```python
from build123d import *

# Parameters (mm, degrees)
BOSS_EXTRUDE1_DEPTH   = 14.2875
F_4_CLEARANCE_HOLE1_D = 3.2639
BOSS_EXTRUDE2_START   = 3.175
SKETCH6_R             = 3.175
SKETCH6_R_2           = 1.63195
BOSS_EXTRUDE2_DEPTH   = 3.175
FILLET1_R             = 3.175
F_2_CLEARANCE_HOLE2_D = 2.4384


with BuildPart() as part:
    # Sketch2 → Boss-Extrude1 (new, symmetric)
    with BuildSketch(Plane.XY):
        Polygon((-14.2875, 0), (-14.2875, 5.08), (-4.5, 5.08), (-4.5, 2.54), (4.5, 2.54), (4.5, 5.08), (14.2875, 5.08), (14.2875, 0), align=None)
    extrude(amount=BOSS_EXTRUDE1_DEPTH, both=True)

    # #4 Clearance Hole1 (through all)
    with Locations(Plane(origin=(0, 5.08, 0), x_dir=(1, 0, 0), z_dir=(0, 1, 0))):
        with Locations((-11.1125, 11.1125), (11.1125, -11.1125), (11.1125, 11.1125), (-11.1125, -11.1125)):
            Hole(F_4_CLEARANCE_HOLE1_D / 2)

    # Sketch6 → Boss-Extrude2 (add)
    # profile 1 of 4: a face of its own
    with BuildSketch(Plane.XZ.offset(BOSS_EXTRUDE2_START)):
        with Locations(Location((-11.1125, 11.1125, 0), (0, 0, 180))):
            Circle(SKETCH6_R)
        with Locations(Location((-11.1125, 11.1125, 0), (0, 0, 90))):
            Circle(SKETCH6_R_2, mode=Mode.SUBTRACT)
    # profile 2 of 4: a face of its own
    with BuildSketch(Plane.XZ.offset(BOSS_EXTRUDE2_START)):
        with Locations((11.1125, 11.1125)):
            Circle(SKETCH6_R)
        with Locations(Location((11.1125, 11.1125, 0), (0, 0, 90))):
            Circle(SKETCH6_R_2, mode=Mode.SUBTRACT)
    # profile 3 of 4: a face of its own
    with BuildSketch(Plane.XZ.offset(BOSS_EXTRUDE2_START)):
        with Locations((11.1125, -11.1125)):
            Circle(SKETCH6_R)
        with Locations(Location((11.1125, -11.1125, 0), (0, 0, 90))):
            Circle(SKETCH6_R_2, mode=Mode.SUBTRACT)
    # profile 4 of 4: a face of its own
    with BuildSketch(Plane.XZ.offset(BOSS_EXTRUDE2_START)):
        with Locations(Location((-11.1125, -11.1125, 0), (0, 0, 180))):
            Circle(SKETCH6_R)
        with Locations(Location((-11.1125, -11.1125, 0), (0, 0, 90))):
            Circle(SKETCH6_R_2, mode=Mode.SUBTRACT)
    extrude(amount=-BOSS_EXTRUDE2_DEPTH)

    # Fillet1
    fillet1_edges = [part.edges().sort_by_distance(p)[0] for p in [
        (-14.2875, 2.54, -14.2875),
        (-14.2875, 2.54, 14.2875),
        (14.2875, 2.54, -14.2875),
        (14.2875, 2.54, 14.2875),
    ]]
    fillet(fillet1_edges, radius=FILLET1_R - 0.0001)  # a hair under: the kernel refuses the full size

    # #2 Clearance Hole2 (through all)
    with Locations(Plane(origin=(0, 2.54, 0), x_dir=(1, 0, 0), z_dir=(0, 1, 0))):
        with Locations((-2.999999969, 5.999999938), (2.999999969, -5.999999938), (2.999999969, 5.999999938), (-2.999999969, -5.999999938)):
            Hole(F_2_CLEARANCE_HOLE2_D / 2)


solid = part.part
```
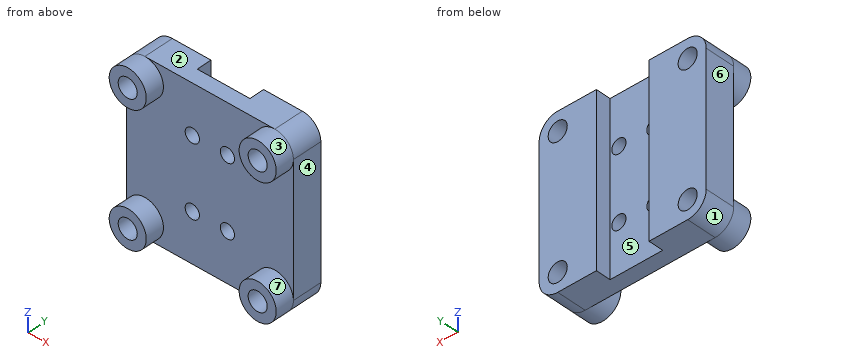
Check sheet for the modelled part. Datum: model origin and axes. Units: mm. Face numbers are marked on the shaded views. A direction names the side the tool comes from. Coordinates: 2 decimals unless noted, no trailing zeros. Write each loop counter-clockwise with the first axis right and the second up, starting at its lowest first coordinate (ties: lowest second). Pieces come first, ordered by that corner, then holes. Notation, with made-up numbers: M 30,9 L 79,9 A23 ccw 79,33 Z; hole C -29.75,-11 d9. An arc over 180 degrees is marked long. Write item = value, one per line. Start each with the question number.
1. Sectioned sample at A-A (y = -0.5). State how many separate pieces and enclosed holes the cut face has, then the cut area to 3 significant figures.
2. Thickness scan on probe 1 along Z at (x, y) = (-3, 0.65); probe 2 along X at (y, z) = (2.75, 1.75); probe 3 along X at (y, z) = (-2.5, -10). Record the ranges inside material, lowest first.
3. Sectioned sample at C-C (x = -2.25). Record the cut outline in (y, z).
4. Sectioned sample at D-D (z = 2.25). Record the cut outline in (x, y).
5. Tool access check on the marked faces 5, 6 and 7. Record the directions out of +Z, -Z, +X, -X, +Y, -Y that give a thin tool (end or side, any length) a straight path to the whole face; none if there is none.
6. Sectioned sample at B-B (z = 6). Record the cut outline in (x, y), then the cut area to 3 significant figures.
7. Mould release check, pull along X, two halves, no side actions. Record for the marked faces 1, 2, 3 and 4: pulls with the +X half, pulls with the -X half, needs draft (parallel to the pull), parting line crosses it, or undercut.
8. Go/stop test with flat-tipped pins: pin 1 (2.5 mm diameter, centred on x = 0, z = 2, fed in from +Y); pin 2 (3 mm diameter, centred on x = -3, z = 6, fed in from -Y); pin 3 (1.5 mm diameter, centred on x = 3, z = 6, fed in from +Y). Record where each tip stops, or that it passes through.
The answers:
q1.separate_pieces = 4
q1.enclosed_holes = 4
q1.area = 93.2 mm²
q2.probe_1 = -14.29 to -7.22, -4.78 to 4.78, 7.22 to 14.29
q2.probe_2 = -14.29 to -4.5, 4.5 to 14.29
q2.probe_3 = -14.09 to -12.31, -9.92 to -8.14, 8.14 to 9.92, 12.31 to 14.09
q3.outline = M 0,-14.29 L 2.54,-14.29 L 2.54,-6.96 L 0,-6.96 Z; M 0,-5.04 L 2.54,-5.04 L 2.54,5.04 L 0,5.04 Z; M 0,6.96 L 2.54,6.96 L 2.54,14.29 L 0,14.29 Z
q4.outline = M -14.29,0 L 14.29,0 L 14.29,5.08 L 4.5,5.08 L 4.5,2.54 L -4.5,2.54 L -4.5,5.08 L -14.29,5.08 Z
q5.face_5 = +Z, -Z, +Y
q5.face_6 = +Z, -Z, -X, +Y, -Y
q5.face_7 = -Y
q6.outline = M -14.29,0 L -4.22,0 L -4.22,2.54 L -4.5,2.54 L -4.5,5.08 L -14.29,5.08 Z; M -1.78,0 L 1.78,0 L 1.78,2.54 L -1.78,2.54 Z; M 4.22,0 L 14.29,0 L 14.29,5.08 L 4.5,5.08 L 4.5,2.54 L 4.22,2.54 Z
q6.area = 110 mm²
q7.face_1 = pulls with the -X half
q7.face_2 = needs draft
q7.face_3 = undercut
q7.face_4 = pulls with the +X half
q8.pin_1 = 2.54
q8.pin_2 = 0
q8.pin_3 = through
